```python
from build123d import *

# Parameters (mm, degrees)
CHANFREIN1_SIZE = 1
CONG_1_R        = 2
CHANFREIN2_SIZE = 1


with BuildPart() as part:
    # Esquisse1 → Révolution1 (revolve)
    with BuildSketch(Plane.XY):
        with BuildLine():
            Line((0, -73.055180274), (-15, -73.055180274))
            Line((-15, -73.055180274), (-15, -69.055180274))
            Line((-15, -69.055180274), (-13.5, -69.055180274))
            Line((-13.5, -69.055180274), (-13.5, -62.055180274))
            Line((-13.5, -62.055180274), (-15, -62.055180274))
            Line((-15, -62.055180274), (-15, -36.055180274))
            Line((-15, -36.055180274), (-19, -33.055180274))
            Line((-19, -33.055180274), (-19, 2.944819726))
            Line((-19, 2.944819726), (-25, 2.944819726))
            Line((-25, 2.944819726), (-25, 16.944819726))
            add(Edge.make_bspline(
                [(-25, 16.944819726), (-19.244550807, 23.982210742), (-19, 32.642645103)],
                knots=[0, 0, 0, 1, 1, 1], degree=2))
            Line((-19, 32.642645103), (-19, 37.642645103))
            Line((-19, 37.642645103), (-10, 53.642645103))
            Line((-10, 53.642645103), (-8.75, 53.642645103))
            add(Edge.make_bspline(
                [(-8.75, 53.642645103), (-8.046565442, 55.307116929), (0, 65.944819726)],
                knots=[0, 0, 0, 1, 1, 1], degree=2))
            Line((0, 65.944819726), (0, -73.055180274))
        make_face()
    revolve(axis=Axis((0, 65.944819726, 0), (0, -1, 0)))

    # Chanfrein1
    chanfrein1_edges = [part.edges().sort_by_distance(p)[0] for p in [
        (25, 2.944819726, 0),
    ]]
    chamfer(chanfrein1_edges, length=CHANFREIN1_SIZE)

    # Congé1
    cong_1_edges = [part.edges().sort_by_distance(p)[0] for p in [
        (19, 2.944819726, 0),
    ]]
    fillet(cong_1_edges, radius=CONG_1_R)

    # Chanfrein2
    chanfrein2_edges = [part.edges().sort_by_distance(p)[0] for p in [
        (15, -73.055180274, 0),
    ]]
    chamfer(chanfrein2_edges, length=CHANFREIN2_SIZE)


solid = part.part
```
Design review of the part built by this model. Coordinates are the model's own, in mm. A direction names the side the tool comes from. Round coordinates to 2 decimals unless told otherwise and drop trailing zeros. Write each loop counter-clockwise with the first axis right and the second up, starting at its lowest first coordinate (ties: lowest second). Pieces come first, ordered by that corner, then holes.
Item 1: Clearance check with flat-ended pins moving along their axes: pin 1 Ø1.5 at (x, z) = (17, -14.5) entering from -Y; pin 2 Ø5 at (x, z) = (-8.5, 0.5) entering from +Y; pin 3 Ø8 at (x, y) = (-9, 0) entering from -Z. State where each tip first meets the part, or that it passes through.
Item 2: The part is to be moulded in two halves that separate along Y. For faces 1 (the cylindrical face through (2.93, -65.51, 13.18)), 2 (the cylindrical face through (-23.846, 10.536, -7.509)), 3 (the conical face through (-10.565, 51.088, 4.38)), 4 (the conical face through (-8.198, -35.868, -12.859)), say which applies: +Y half, -Y half, draft (parallel to the pull), parting line (faces both ways), or undercut.
Item 3: For faces 5 (the flat face through (-11.18, -62.055, -7.85)), 6 (the cylindrical face through (14.985, -70.534, -0.66)), 7 (the flat face through (0, -73.055, 0)), 8 (the cylindrical face through (-8.767, 35.178, 16.856)), list the 3-axis set-ups (+Z, -Z, +X, -X, +Y, -Y) from which the entire face can be reached by the end or side of a thin tool; tool diameter is ignored.
Item 4: We need section A-A on y = 49. Write out the cut boundary in (x, z), and give its area (3 significant figures).
Item 5: For probe 1 along Y at (x, z) = (12, 7.5); probe 2 along Z at (x, y) = (0, -47.5); probe 3 along X at (y, z) = (10.5, 8), list the stretches that pass through material, from the lowest coordinate up.
Returned:
1. pin 1: stops at y = 2.94
1. pin 2: stops at y = 57.83
1. pin 3: stops at z = -23.62
2. face 1: undercut
2. face 2: draft
2. face 3: +Y half
2. face 4: -Y half
3. face 5: none
3. face 6: -Y
3. face 7: +Z, -Z, +X, -X, -Y
3. face 8: +Y
4. outline: circle Ø25.22 at (0, 0)
4. area: 500 mm2
5. probe 1: y = -72.9 to -69.06, -62.06 to 46.26
5. probe 2: z = -15 to 15
5. probe 3: x = -23.69 to 23.69
